The model under review builds one solid part; all positions refer to its coordinate system, in mm. A direction names the side the tool comes from. Coordinates: 2 decimals unless noted, no trailing zeros. Order: outer loops, then holes, each group sorted by start corner. A loop starts at its lowest first (then second) coordinate and runs counter-clockwise, first axis right, second up. Notation, with made-up numbers: (19, -25.5) - (58, -25.5) arc R31 ccw to (58, -0.5) - close; hole circle Ø6 at (38.25, 13). An arc over 180 degrees is marked (long way). Answer in a Markdown table with one row per item.
```python
from build123d import *

# Parameters (mm, degrees)
SKETCH_R        = 70
SKETCH_R_2      = 57.25
PAD_DEPTH       = 15
SKETCH001_R     = 4
SKETCH002_W     = 40
SKETCH002_H     = 40
PAD001_DEPTH    = 5
SKETCH003_R     = 2.5
POCKET_DEPTH    = 5
FILLET_R        = 18
FILLET001_R     = 11
SKETCH004_R     = 58
POCKET001_DEPTH = 15.001
SKETCH005_R     = 71
POCKET002_DEPTH = 7
SKETCH006_R     = 4


with BuildPart() as part:
    # Sketch → Pad (new body)
    with BuildSketch(Plane.XY):
        Circle(SKETCH_R)
        Circle(SKETCH_R_2, mode=Mode.SUBTRACT)
    extrude(amount=PAD_DEPTH)

    # Sketch001 → Groove (revolve, cut)
    with BuildSketch(Plane.XZ):
        with Locations((63.625, 16)):
            Circle(SKETCH001_R)
    revolve(axis=Axis((0, 0, 0), (0, 0, 1)), mode=Mode.SUBTRACT)

    # Sketch002 (on Face2 of Groove) → Pad001 (join)
    with BuildSketch(Plane(origin=(0, 0, 0), x_dir=(1, 0, 0), z_dir=(0, 0, -1))):
        with Locations((82, 0)):
            Rectangle(SKETCH002_W, SKETCH002_H)
        with Locations((-82, 0)):
            Rectangle(SKETCH002_W, SKETCH002_H)
        with Locations((0, 82)):
            Rectangle(SKETCH002_W, SKETCH002_H)
        with Locations((0, -82)):
            Rectangle(SKETCH002_W, SKETCH002_H)
    extrude(amount=-PAD001_DEPTH)

    # Sketch003 (on Face13 of Pad001) → Pocket (cut)
    with BuildSketch(Plane.XY.offset(5)):
        with Locations((-86.25, 0)):
            Circle(SKETCH003_R)
        with Locations((0, -86.25)):
            Circle(SKETCH003_R)
        with Locations((86.25, 0)):
            Circle(SKETCH003_R)
        with Locations((0, 86.25)):
            Circle(SKETCH003_R)
    extrude(amount=-POCKET_DEPTH, mode=Mode.SUBTRACT)

    # Fillet
    fillet_edges = [part.edges().sort_by_distance(p)[0] for p in [
        (-20, 102, 2.5),
        (20, 102, 2.5),
        (102, 20, 2.5),
        (102, -20, 2.5),
        (20, -102, 2.5),
        (-20, -102, 2.5),
        (-102, -20, 2.5),
        (-102, 20, 2.5),
    ]]
    fillet(fillet_edges, radius=FILLET_R)

    # Fillet001
    fillet001_edges = [part.edges().sort_by_distance(p)[0] for p in [
        (67.082039, 20, 2.5),
        (20, 67.082039, 2.5),
        (-20, 67.082039, 2.5),
        (-67.082039, 20, 2.5),
        (-67.082039, -20, 2.5),
        (-20, -67.082039, 2.5),
        (20, -67.082039, 2.5),
        (67.082039, -20, 2.5),
    ]]
    fillet(fillet001_edges, radius=FILLET001_R)

    # Sketch004 (on Face41 of Fillet001) → Pocket001 (cut, through all)
    with BuildSketch(Plane.XY.offset(15)):
        Circle(SKETCH004_R)
    extrude(amount=-POCKET001_DEPTH, mode=Mode.SUBTRACT)

    # Sketch005 (on Face38 of Pocket001) → Pocket002 (cut)
    with BuildSketch(Plane.XY.offset(15)):
        Circle(SKETCH005_R)
    extrude(amount=-POCKET002_DEPTH, mode=Mode.SUBTRACT)

    # Sketch006 → Groove001 (revolve, cut)
    with BuildSketch(Plane.XZ):
        with Locations((63.625, 9)):
            Circle(SKETCH006_R)
    revolve(axis=Axis((0, 0, 0), (0, 0, 1)), mode=Mode.SUBTRACT)


solid = part.part
```
Item 1: To check wall thickness, follow line 1 (X direction, y = 37.5, z = 7.5); line 2 (X direction, y = -18, z = 5.5); line 3 (Y direction, x = 27.5, z = 5.5). State the ranges of each line that lie inside material, in increasing order. Write a range as from..to.
Check values:
| item | result |
|---|---|
| line 1 | -59.11..-55.92, -46.73..-44.25, 44.25..46.73, 55.92..59.11 |
| line 2 | -67.65..-63.04, -59..-55.14, 55.14..59, 63.04..67.65 |
| line 3 | -64.37..-59.52, -55.22..-51.07, 51.07..55.22, 59.52..64.37 |
Item 2: Tool access review of faces 1 (the face through (79, 20, 2)), 2 (the face through (20, -79, 2)), 3 (the face through (32.301, -62.102, 4.833)): name each direction out of +Z, -Z, +X, -X, +Y, -Y from which nothing blocks a thin tool from reaching the whole face with its end or side.
Check values:
| item | result |
|---|---|
| face 1 | +Z, -Z, +X, +Y |
| face 2 | +Z, -Z, +X, -Y |
| face 3 | +Z |
Item 3: We need section B-B, the plane z = 2. State how many separate pieces and enclosed holes the cut face has, then the cut area to 3 significant figures.
Check values:
| item | result |
|---|---|
| separate pieces | 1 |
| enclosed holes | 5 |
| area | 9,550 mm^2 |
Item 4: We need section A-A, the plane y = 79.5. Write out the cut boundary in (x, z).
Check values:
| item | result |
|---|---|
| outline | (-20, 0) - (20, 0) - (20, 5) - (-20, 5) - close |
Item 5: Clearance check with flat-ended pins moving along their axes: pin 1 Ø1.5 at (y, z) = (-81.5, 2.5) entering from +X; pin 2 Ø11 at (x, y) = (-10.5, -75) entering from +Z; pin 3 Ø4 at (y, z) = (80.5, 3) entering from -X. State where each tip first meets the part, or that it passes through.
Check values:
| item | result |
|---|---|
| pin 1 | x = 20 |
| pin 2 | z = 5 |
| pin 3 | x = -20 |
